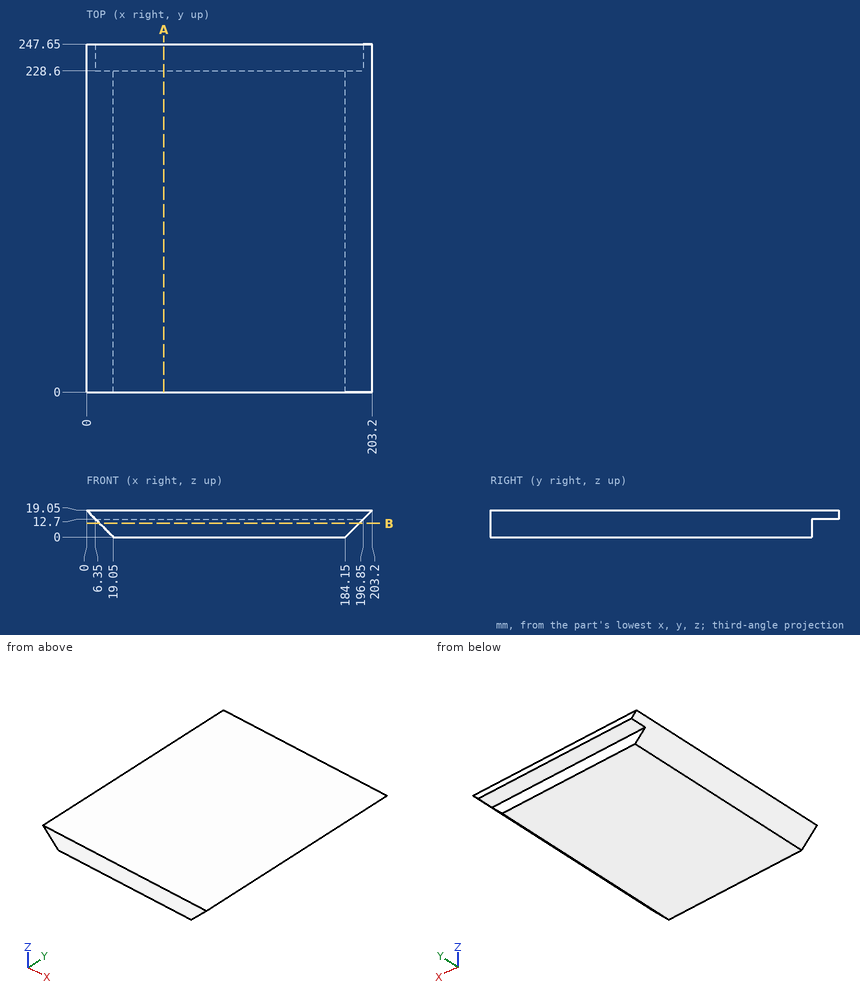
Answer from the drawing. Dimensions are ordinates in mm from the lowest x, y and z of the part. Coordinates: 2 decimals unless noted, no trailing zeros. Write each loop counter-clockwise with the first axis right and the second up, starting at its lowest first coordinate (ties: lowest second). Pieces come first, ordered by that corner, then holes. Notation, with made-up numbers: M 2,-12 L 41,-12 A16 ccw 41,4 Z; hole C 82,61.5 d7. An arc over 180 degrees is marked long. Use one line per item in the form item = value. Start each with the question number.
1. Each of these flat-tipped pins is pushed along its axis until it touches: P1, Ø15, axis at x = 117, y = 233.5, coming from the -Z side; P2, Ø1.5, axis at y = 195.5, z = 6.5, coming from the +X side; P3, Ø6, axis at y = 48.5, z = 9.5, coming from the +X side; P4, Ø6, axis at y = 155, z = 2.5, coming from the -X side. Where does it stop, or does it pass through?
2. Straight lines are drawn through the part: probe 1 along Y at (x, z) = (32, 10.5); probe 2 along X at (y, z) = (223, 4.75); probe 3 along X at (y, z) = (110, 13). For each, find the intervals that lie inside material, in ascending order. Write a range as from..to.
3. The part is cut by section A-A (x = 55). Give the vertices of the cut face in (y, z), plus the area to 3 significant figures.
4. The part is cut by section B-B (z = 9.75). Give the vertices of the cut face in (x, y), plus the area to 3 significant figures.
Evaluation:
q1.P1 = 0
q1.P2 = 191.4
q1.P3 = 196.65
q1.P4 = 13.55
q2.probe_1 = 0..228.6
q2.probe_2 = 14.3..188.9
q2.probe_3 = 6.05..197.15
q3.outline = M 0,0 L 228.6,0 L 228.6,12.7 L 247.65,12.7 L 247.65,19.05 L 0,19.05 Z
q3.area = 4,480 mm^2
q4.outline = M 9.3,0 L 193.9,0 L 193.9,228.6 L 9.3,228.6 Z
q4.area = 42,200 mm^2
